Model file for the job. Use its own axes, mm. A direction names the side the tool comes from. Round coordinates to 2 decimals unless told otherwise and drop trailing zeros. Order: outer loops, then holes, each group sorted by start corner. A loop starts at its lowest first (then second) coordinate and runs counter-clockwise, first axis right, second up. Notation, with made-up numbers: M -9.75,13 L 25.25,13 A29 cw 25.25,36 Z; hole C 27.25,44.25 d1. An arc over 180 degrees is marked long. Return JSON: item names as keys, results as strings. Group by question number.
Item 1: Slice it at D-D on x = -19. Write the cut outline in (y, z), then the cut area to 3 significant figures.
Item 2: Which spindle directions (+Z, -Z, +X, -X, +Y, -Y) get a long thin tool onto all of the face, cutting with end or side? Do faces 5 (the face through (-5.172, -43.042, 3.944)), 6 (the face through (0, -36.5, 2)). Say none if no direction does.
Item 3: Pin check, flat tips, straight feed: pin 1 Ø1.2 at (y, z) = (-37.5, 3.5) entering from -X; pin 2 Ø2 at (x, z) = (-39, 5) entering from +Y; pin 3 Ø1 at (x, z) = (14.5, 6.5) entering from -Y. Stop position of each tip, or through.
Item 4: Slice it at B-B on z = 6.5. Give the number of separate pieces and of enclosed holes in the cut face, then the cut area to 3 significant figures.
Item 5: Pull direction Y, two halves, no side cores. Call faces 1 (the face through (-46, 0, 4)), 2 (the face through (-5.22, 42.96, 3.94)), 3 (the face through (25.594, -26.023, 3.944)), 4 (the face through (-38.274, 3.045, 2.465)): pulls with the +Y half, pulls with the -Y half, needs draft (parallel to the pull), parting line crosses it, or undercut.
Item 6: Probe line 1 along Y through (x, z) = (0, 2.75); line 2 along Y through (x, z) = (-40, 7.1). List the from-to ranges inside material, lowest first.
Item 7: Slice it at A-A on y = 0. Write the cut outline in (x, z).
from build123d import *

# Parameters (mm, degrees)
SKETCH_R              = 36.5
SKETCH_R_2            = 30.5
PAD_DEPTH             = 8
SKETCH002_R           = 2.1
PAD001_DEPTH          = 8
POLARPATTERN_COUNT    = 4
POCKET001_DEPTH       = 5
POLARPATTERN001_COUNT = 4


with BuildPart() as part:
    # Sketch → Pad (new body)
    with BuildSketch(Plane.XY):
        Circle(SKETCH_R)
        Circle(SKETCH_R_2, mode=Mode.SUBTRACT)
    extrude(amount=PAD_DEPTH)

    # Sketch002 (on Face3 of Pad) → Pad001 (join)
    with BuildSketch(Plane(origin=(0, 0, 0), x_dir=(1, 0, 0), z_dir=(0, 0, -1))):
        with BuildLine():
            Line((-40, 6.928203), (-46, 3.464102))
            Line((-46, 3.464102), (-46, -3.464102))
            Line((-46, -3.464102), (-40, -6.928203))
            Line((-40, -6.928203), (-35.836434, -6.928203))
            ThreePointArc((-35.836434, 6.928203), (-36.5, 0), (-35.836434, -6.928203))
            Line((-40, 6.928203), (-35.836434, 6.928203))
        make_face()
        with Locations((-40, 0)):
            Circle(SKETCH002_R, mode=Mode.SUBTRACT)
    pad001 = extrude(amount=-PAD001_DEPTH)

    # PolarPattern: Pad001 ×4 about axis
    polarpattern_axis = Axis((0, 0, 0), (0, 0, -1))
    for i in range(1, POLARPATTERN_COUNT):
        add(pad001.rotate(polarpattern_axis, i * 360 / POLARPATTERN_COUNT))

    # Sketch003 (on Face2 of PolarPattern) → Pocket001 (cut)
    with BuildSketch(Plane(origin=(0, 0, 0), x_dir=(1, 0, 0), z_dir=(0, 0, -1))):
        Polygon((-36.5, 2.020726), (-40, 4.041452), (-43.5, 2.020726), (-43.5, -2.020726), (-40, -4.041452), (-36.5, -2.020726), align=None)
    pocket001 = extrude(amount=-POCKET001_DEPTH, mode=Mode.SUBTRACT)

    # PolarPattern001: Pocket001 ×4 about axis
    polarpattern001_axis = Axis((0, 0, 0), (0, 0, -1))
    for i in range(1, POLARPATTERN001_COUNT):
        add(pocket001.rotate(polarpattern001_axis, i * 360 / POLARPATTERN001_COUNT), mode=Mode.SUBTRACT)


solid = part.part
Output values:
{
 "1": {"outline": "M -31.16,0 L -23.86,0 L -23.86,8 L -31.16,8 Z; M 23.86,0 L 31.16,0 L 31.16,8 L 23.86,8 Z", "area": "117 mm²"},
 "2": {"face 5": "+Z, -Z, -X, -Y", "face 6": "-Z"},
 "3": {"pin 1": "x = -6.93", "pin 2": "y = 6.93", "pin 3": "y = -33.71"},
 "4": {"separate pieces": "1", "enclosed holes": "5", "area": "1,660 mm²"},
 "5": {"face 1": "needs draft", "face 2": "pulls with the +Y half", "face 3": "pulls with the -Y half", "face 4": "undercut"},
 "6": {"line 1": "-46 to -43.5, -36.5 to -30.5, 30.5 to 36.5, 43.5 to 46", "line 2": "-6.93 to -2.1, 2.1 to 6.93"},
 "7": {"outline": "M -46,0 L -43.5,0 L -43.5,5 L -42.1,5 L -42.1,8 L -46,8 Z; M -37.9,5 L -36.5,5 L -36.5,0 L -30.5,0 L -30.5,8 L -37.9,8 Z; M 30.5,0 L 36.5,0 L 36.5,5 L 37.9,5 L 37.9,8 L 30.5,8 Z; M 42.1,5 L 43.5,5 L 43.5,0 L 46,0 L 46,8 L 42.1,8 Z"}
}
